Check sheet for the drawn part. Datum: minimum x, y, z corner. Units: mm. Round coordinates to 2 decimals unless told otherwise and drop trailing zeros. Loops run counter-clockwise (first coordinate to the right, second up) from the corner with the lowest first, then second, coordinate; pieces in that order, holes last. Notation, with made-up numbers: (5.25, 38.25) -> (16.25, 38.25) arc R11 ccw to (16.25, 42.25) -> close; hole circle Ø9 at (32.5, 35.5). An arc over 180 degrees is marked (long way). Write item = value, one per line. Start each with the question number.
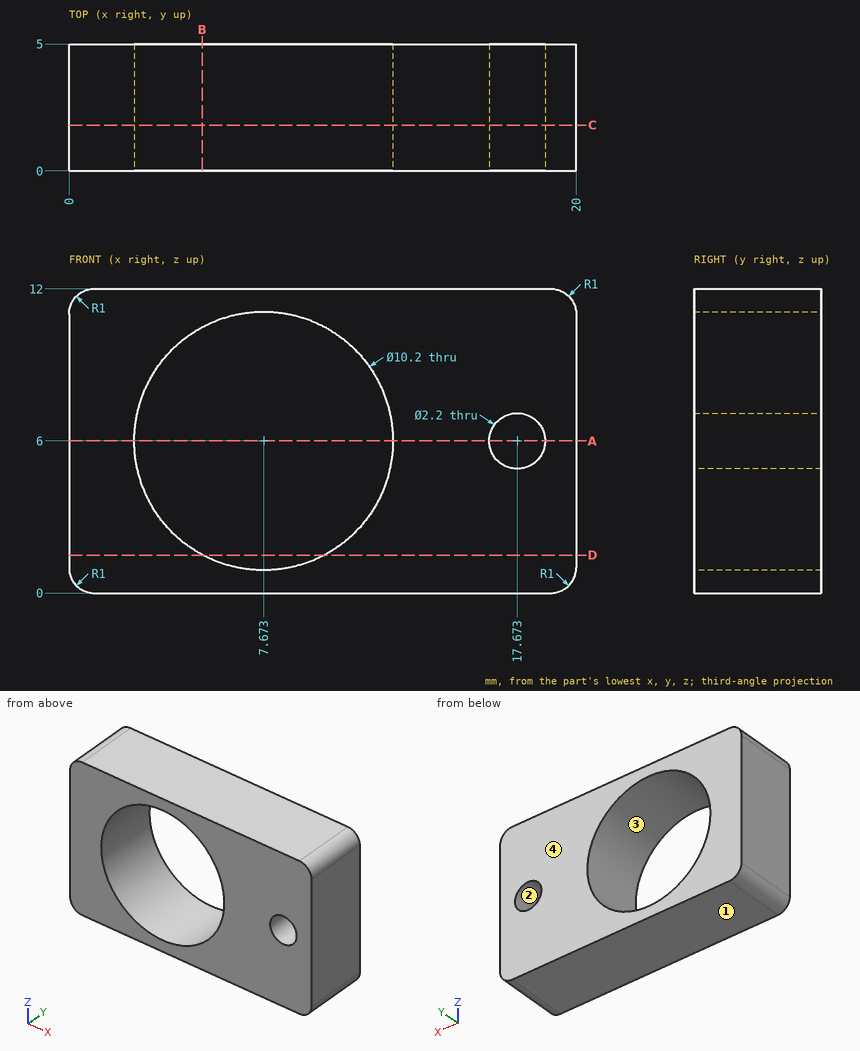
(1) Draft check along Z on the marked faces 1, 2, 3 and 4. Enter one of: +Z half, -Z half, draft (parallel to the pull), parting line (faces both ways), or undercut.
(2) Section check A-A on z = 6. Enter the section's corners in (x, y).
(3) Section check B-B on x = 5.25. Enter the section's corners in (y, z), then the cut area to 3 significant figures.
(4) Section check D-D on z = 1.5. Enter the section's corners in (x, y).
(5) Section check C-C on y = 1.8. Enter the section's corners in (x, z).
(6) Scan lines: line 1 (X direction, y = 3.75, z = 6); line 2 (Z direction, x = 12, y = 2.85); line 3 (Z direction, x = 5.75, y = 4.2). Record each from-to range of solid material in increasing order. Write a range as [from, to].
Computed values:
q1.face_1 = -Z half
q1.face_2 = undercut
q1.face_3 = undercut
q1.face_4 = draft
q2.outline = (0, 0) -> (2.57, 0) -> (2.57, 5) -> (0, 5) -> close; (12.77, 0) -> (16.57, 0) -> (16.57, 5) -> (12.77, 5) -> close; (18.77, 0) -> (20, 0) -> (20, 5) -> (18.77, 5) -> close
q3.outline = (0, 0) -> (5, 0) -> (5, 1.51) -> (0, 1.51) -> close; (0, 10.49) -> (5, 10.49) -> (5, 12) -> (0, 12) -> close
q3.area = 15.1 mm²
q4.outline = (0, 0) -> (5.27, 0) -> (5.27, 5) -> (0, 5) -> close; (10.07, 0) -> (20, 0) -> (20, 5) -> (10.07, 5) -> close
q5.outline = (0, 1) arc R1 ccw to (1, 0) -> (19, 0) arc R1 ccw to (20, 1) -> (20, 11) arc R1 ccw to (19, 12) -> (1, 12) arc R1 ccw to (0, 11) -> close; hole circle Ø10.2 at (7.67, 6); hole circle Ø2.2 at (17.67, 6)
q6.line_1 = [0, 2.57], [12.77, 16.57], [18.77, 20]
q6.line_2 = [0, 3.3], [8.7, 12]
q6.line_3 = [0, 1.28], [10.72, 12]
